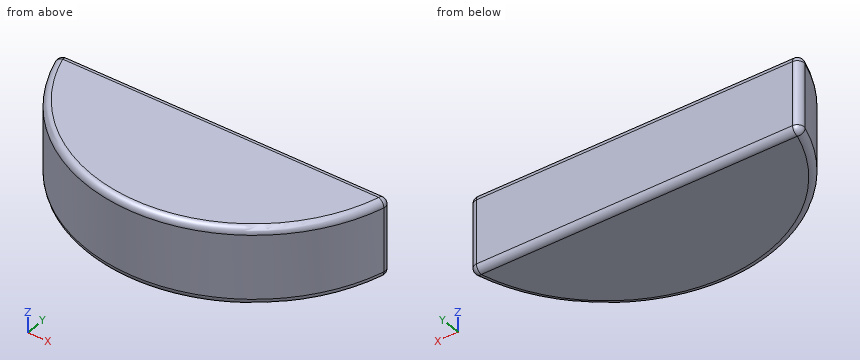
```python
from build123d import *

# Parameters (mm, degrees)
EXTRUDE1_DEPTH = 1.5
FILLET1_R      = 0.254


with BuildPart() as part:
    # Sketch1 → Extrude1 (new body, symmetric)
    with BuildSketch(Plane.XY):
        with BuildLine():
            Line((-6.325, -1.498123827), (6.325, -1.498123827))
            ThreePointArc((6.325, -1.498123827), (0, -6.5), (-6.325, -1.498123827))
        make_face()
    extrude(amount=EXTRUDE1_DEPTH, both=True)

    # Fillet1
    fillet1_edges = [part.edges().sort_by_distance(p)[0] for p in [
        (0, -1.498123827, -1.5),
        (0, -6.5, -1.5),
        (0, -6.5, 1.5),
        (-6.325, -1.498123827, 0),
        (6.325, -1.498123827, 0),
        (0, -1.498123827, 1.5),
    ]]
    fillet(fillet1_edges, radius=FILLET1_R)


solid = part.part
```
Could you check a few things on this model? Use its own coordinates, in mm. Round coordinates to 2 decimals unless told otherwise and drop trailing zeros. Order: outer loops, then holes, each group sorted by start corner. A loop starts at its lowest first (then second) coordinate and runs counter-clockwise, first axis right, second up. Notation, with made-up numbers: M 45,25 L 81,25 A19 ccw 81,36 Z; hole C -2,86.5 d5. An arc over 180 degrees is marked long. One line per question, with ' | ' between items. Start each with the question number.
(1) Please list where these lines run through material, in increasing order: line 1 along X through (y, z) = (-4.95, 0.5); line 2 along Z through (x, y) = (-5.5, -3.35); line 3 along Y through (x, z) = (2.25, 0.15).
(2) For P1, Ø1, axis at y = -3, z = 0.5, coming from the +X side, with a flat end and sliding along its axis, tell me the tip position at first contact or that it passes through.
(3) Suppose I cut it at A-A on z = 1.1. List the corners of the cut face in (x, y) for me.
Geometry results:
1) line 1: -4.21 to 4.21 | line 2: -1.41 to 1.41 | line 3: -6.1 to -1.5
2) P1: x = 6
3) outline: M -6.24,-1.82 A6.5 ccw 6.24,-1.82 A0.25 ccw 6,-1.5 L -6,-1.5 A0.25 ccw Z
